from build123d import *

# Parameters (mm, degrees)
EXTRUDE_1_DEPTH   = 25
EXTRUDE_1_2_DEPTH = 25
EXTRUDE_1_3_DEPTH = 25
EXTRUDE_1_4_DEPTH = 25
EXTRUDE_1_5_DEPTH = 25
EXTRUDE_1_6_DEPTH = 25
SKETCH_2_R        = 28.5
EXTRUDE_2_DEPTH   = 5
EXTRUDE_4_DEPTH   = 5


with BuildPart() as part:
    # Sketch 1 → Extrude 1 (new body)
    with BuildSketch(Plane(origin=(0, 0, 0), x_dir=(1, 0, 0), z_dir=(0, 1, 0))):
        Polygon((4.794019272, 13.629956631), (4.962963937, 11.898177863), (6.547200676, 11.178598851), (7.96249275, 12.190798607), (7.793548085, 13.922577374), (6.209311346, 14.642156386), align=None)
    extrude(amount=EXTRUDE_1_DEPTH)



with BuildPart() as body_2:
    # Sketch 1 → Extrude 1 2 (new body)
    with BuildSketch(Plane(origin=(0, 0, 0), x_dir=(1, 0, 0), z_dir=(0, 1, 0))):
        Polygon((15.954079735, 0.21187806), (15.78513507, 1.943656828), (14.200898331, 2.66323584), (12.785606257, 1.651036084), (12.954550922, -0.080742684), (14.538787661, -0.800321696), align=None)
    extrude(amount=EXTRUDE_1_2_DEPTH)


with BuildPart() as body_3:
    # Sketch 1 → Extrude 1 3 (new body)
    with BuildSketch(Plane(origin=(0, 0, 0), x_dir=(1, 0, 0), z_dir=(0, 1, 0))):
        Polygon((8.16053165, -13.710699314), (9.575823724, -12.698499559), (9.406879059, -10.966720791), (7.82264232, -10.247141779), (6.407350246, -11.259341535), (6.576294911, -12.991120302), align=None)
    extrude(amount=EXTRUDE_1_3_DEPTH)


with BuildPart() as body_4:
    # Sketch 1 → Extrude 1 4 (new body)
    with BuildSketch(Plane(origin=(0, 0, 0), x_dir=(1, 0, 0), z_dir=(0, 1, 0))):
        Polygon((-7.793548085, -13.922577374), (-6.209311346, -14.642156386), (-4.794019272, -13.629956631), (-4.962963937, -11.898177863), (-6.547200676, -11.178598851), (-7.96249275, -12.190798607), align=None)
    extrude(amount=EXTRUDE_1_4_DEPTH)


with BuildPart() as body_5:
    # Sketch 1 → Extrude 1 5 (new body)
    with BuildSketch(Plane(origin=(0, 0, 0), x_dir=(1, 0, 0), z_dir=(0, 1, 0))):
        Polygon((-12.785606257, -1.651036084), (-12.954550922, 0.080742684), (-14.538787661, 0.800321696), (-15.954079735, -0.21187806), (-15.78513507, -1.943656828), (-14.200898331, -2.66323584), align=None)
    extrude(amount=EXTRUDE_1_5_DEPTH)


with BuildPart() as body_6:
    # Sketch 1 → Extrude 1 6 (new body)
    with BuildSketch(Plane(origin=(0, 0, 0), x_dir=(1, 0, 0), z_dir=(0, 1, 0))):
        Polygon((-6.576294911, 12.991120302), (-8.16053165, 13.710699314), (-9.575823724, 12.698499559), (-9.406879059, 10.966720791), (-7.82264232, 10.247141779), (-6.407350246, 11.259341535), align=None)
    extrude(amount=EXTRUDE_1_6_DEPTH)


with BuildPart() as part_1:
    add(part.part)

    add(body_2.part)  # Extrude 2 merges body 2

    add(body_3.part)  # Extrude 2 merges body 3

    add(body_4.part)  # Extrude 2 merges body 4

    add(body_5.part)  # Extrude 2 merges body 5

    add(body_6.part)  # Extrude 2 merges body 6
    # Sketch 2 → Extrude 2 (add)
    with BuildSketch(Plane(origin=(0, 0, 0), x_dir=(1, 0, 0), z_dir=(0, 1, 0))):
        with Locations(Location((0, 0, 0), (0, 0, 270))):
            Circle(SKETCH_2_R)
    extrude(amount=-EXTRUDE_2_DEPTH)

    # Sketch 3 → Extrude 4 (add)
    with BuildSketch(Plane(origin=(0, -5, 0), x_dir=(-1, 0, 0), z_dir=(0, -1, 0))):
        Polygon((6.067131278, 3.713249853), (8.603282508, 2.334384279), (11.065490739, 3.841322885), (10.991547739, 6.727127065), (8.455396509, 8.105992639), (5.993188279, 6.599054033), align=None)
        Polygon((0, -7.113248654), (-2.5, -8.556624327), (-2.5, -11.443375673), (0, -12.886751346), (2.5, -11.443375673), (2.5, -8.556624327), align=None)
        Polygon((-6.334313735, 3.236475849), (-6.482151211, 6.119439153), (-9.052789409, 7.432889795), (-11.475590131, 5.863377133), (-11.327752654, 2.980413829), (-8.757114457, 1.666963187), align=None)
    extrude(amount=EXTRUDE_4_DEPTH)


solid = part_1.part
Design review of the part built by this model. Coordinates are the model's own, in mm. A direction names the side the tool comes from. Coordinates: 2 decimals unless noted, no trailing zeros. Order: outer loops, then holes, each group sorted by start corner. A loop starts at its lowest first (then second) coordinate and runs counter-clockwise, first axis right, second up.
Item 1: For line 1 (Y direction, x = 14, z = 5); line 2 (X direction, y = 22, z = -13); line 3 (Z direction, x = 24.5, y = -3), list the stretches that pass through material, from the lowest coordinate up.
Item 2: The part is to be moulded in two halves that separate along X. For faces 1 (the flat face through (13.736, 12.325, 0.435)), 2 (the flat face through (-7.88, 12.32, 13.04)), 3 (the flat face through (10.247, -7.465, -6.659)), 4 (the flat face through (-5.744, 12.325, 11.543)), say which applies: pulls with the +X half, pulls with the -X half, needs draft (parallel to the pull), parting line crosses it, or undercut.
Item 3: Take a section at B-B, the plane z = 25.5. Write out the cut boundary in (x, y).
Item 4: For faces 5 (the flat face through (-9.82, -7.46, -3.08)), 6 (the flat face through (13.5, 12.32, -2.16)), 7 (the flat face through (9.493, 12.325, 11.845)), 8 (the flat face through (-9.741, -7.465, -7.407)), list the 3-axis set-ups (+Z, -Z, +X, -X, +Y, -Y) from which the entire face can be reached by the end or side of a thin tool; tool diameter is ignored.
Item 5: Take a section at C-C, the plane x = -19. Write out the cut boundary in (y, z), then the cut area to 3 significant figures.
Item 6: For pin 1 Ø0.9 at (y, z) = (-7, 9.5) entering from +X; pin 2 Ø3 at (x, z) = (-22.5, -15.5) entering from +Y; pin 3 Ø6 at (y, z) = (1.5, -9) entering from -X, all flat-tipped, find the tip position at first contact; note any pin that passes through.
Item 7: Take a section at A-A, the plane y = 11.5. Count the separate pieces of the cut face and the enclosed holes in it, then the cut area to 3 significant figures.
The answers:
1. line 1: y = -5 to 0
1. line 2: x = -9.15 to -6.6, 4.86 to 7.88
1. line 3: z = -14.56 to 14.56
2. face 1: undercut
2. face 2: pulls with the -X half
2. face 3: pulls with the +X half
2. face 4: undercut
3. outline: (-12.73, -5) - (12.73, -5) - (12.73, 0) - (-12.73, 0) - close
4. face 5: +Z, -X, -Y
4. face 6: -Z, -X, +Y
4. face 7: -Z, +X, +Y
4. face 8: -Z, -X, -Y
5. outline: (-5, -21.24) - (0, -21.24) - (0, 21.24) - (-5, 21.24) - close
5. area: 212 mm2
6. pin 1: stops at x = 2.5
6. pin 2: stops at y = 0
6. pin 3: stops at x = -27.77
7. separate pieces: 6
7. enclosed holes: 0
7. area: 47.2 mm2
